Geometry check sheet. Reference: the model listing, model coordinates, mm. A direction names the side the tool comes from. Give positions to 0.01 mm unless a question says otherwise; leave off trailing zeros. Loops run counter-clockwise (first coordinate to the right, second up) from the corner with the lowest first, then second, coordinate; pieces in that order, holes last. Notation, with made-up numbers: (66, 88) -> (80, 88) arc R21 ccw to (80, 114) -> close; hole circle Ø5 at (32, 8). An arc over 180 degrees is marked (long way). Answer in a Markdown table with one row per item. Add a question column.
```python
from build123d import *

# Parameters (mm, degrees)
SKETCH1_W           = 20
SKETCH1_H           = 38
BOSS_EXTRUDE1_DEPTH = 3
SKETCH2_W           = 10
SKETCH2_H           = 3
CUT_EXTRUDE1_DEPTH  = 3
CUT_EXTRUDE2_DEPTH  = 3


with BuildPart() as part:
    # Sketch1 → Boss-Extrude1 (new body)
    with BuildSketch(Plane(origin=(0, 0, 0), x_dir=(0, 0, -1), z_dir=(1, 0, 0))):
        with Locations((10, 19)):
            Rectangle(SKETCH1_W, SKETCH1_H)
    extrude(amount=BOSS_EXTRUDE1_DEPTH)

    # Sketch2 → Cut-Extrude1 (cut)
    with BuildSketch(Plane(origin=(3, 0, 0), x_dir=(0, 0, -1), z_dir=(1, 0, 0))):
        with Locations((5, 36.5)):
            Rectangle(SKETCH2_W, SKETCH2_H)
        with Locations((5, 1.5)):
            Rectangle(SKETCH2_W, SKETCH2_H)
    extrude(amount=-CUT_EXTRUDE1_DEPTH, mode=Mode.SUBTRACT)

    # Sketch3 → Cut-Extrude2 (cut)
    with BuildSketch(Plane(origin=(3, 0, 0), x_dir=(0, 0, -1), z_dir=(1, 0, 0))):
        Polygon((3.45, 3), (3.45, 5.9), (2.05, 5.9), (2.05, 8.6), (3.45, 8.6), (3.45, 10.3), (6.55, 10.3), (6.55, 8.6), (7.95, 8.6), (7.95, 5.9), (6.55, 5.9), (6.55, 3), align=None)
        Polygon((6.55, 35), (6.55, 32.1), (7.95, 32.1), (7.95, 29.4), (6.55, 29.4), (6.55, 27.7), (3.45, 27.7), (3.45, 29.4), (2.05, 29.4), (2.05, 32.1), (3.45, 32.1), (3.45, 35), align=None)
    extrude(amount=-CUT_EXTRUDE2_DEPTH, mode=Mode.SUBTRACT)


solid = part.part
```
1. Material ranges on L1, parallel to Y at x = 0.55, z = -2.75; L2, parallel to Z at x = 0.8, y = 10; L3, parallel to Z at x = 0.6, y = 31, recorded low to high. Write a range as from..to.
2. Sectioned sample at B-B (z = -7.5). Enter the section's corners in (x, y).
3. Access from +Z, -Z, +X, -X, +Y, -Y to the whole of each face (thin tool, end or side, straight path). Record for faces 1 (the face through (2, 1, -10)), 2 (the face through (1, 0, -15)), 3 (the face through (2, 9, -6.55)), 4 (the face through (2, 8.6, -3)), 5 (the face through (2, 35, -8)).
4. Release check for a two-part mould opening along Y. For faces 6 (the face through (2, 27.7, -5)), 7 (the face through (2, 7, -2.05)), 8 (the face through (2, 4, -6.55)) record: released by +Y, released by -Y, zero draft, split by the parting line, or undercut.
5. Sectioned sample at A-A (y = 7). Enter the section's corners in (x, z), plus the area to 3 significant figures.
6. Sectioned sample at D-D (z = -4.5). Enter the section's corners in (x, y).
7. Gauge pin test, flat ends, axial feed: pin 1 Ø1.4 at (x, y) = (2, 28.5) entering from +Z; pin 2 Ø1.5 at (x, z) = (2, -3) entering from -Y; pin 3 Ø0.7 at (x, z) = (1, -7) entering from +Y. Record the tip position at first contact, or that the pin passes through.
Response:
| question | item | result |
|---|---|---|
| 1 | L1 | y = 3..5.9, 8.6..29.4, 32.1..35 |
| 1 | L2 | z = -20..-6.55, -3.45..0 |
| 1 | L3 | z = -20..-7.95, -2.05..0 |
| 2 | outline | (0, 3) -> (3, 3) -> (3, 5.9) -> (0, 5.9) -> close; (0, 8.6) -> (3, 8.6) -> (3, 29.4) -> (0, 29.4) -> close; (0, 32.1) -> (3, 32.1) -> (3, 35) -> (0, 35) -> close |
| 3 | face 1 | +Z, +X, -X, -Y |
| 3 | face 2 | +Z, -Z, +X, -X, -Y |
| 3 | face 3 | +X, -X, -Y |
| 3 | face 4 | +X, -X |
| 3 | face 5 | +Z, +X, -X, +Y |
| 4 | face 6 | released by +Y |
| 4 | face 7 | undercut |
| 4 | face 8 | zero draft |
| 5 | outline | (0, -20) -> (3, -20) -> (3, -7.95) -> (0, -7.95) -> close; (0, -2.05) -> (3, -2.05) -> (3, 0) -> (0, 0) -> close |
| 5 | area | 42.3 mm2 |
| 6 | outline | (0, 10.3) -> (3, 10.3) -> (3, 27.7) -> (0, 27.7) -> close |
| 7 | pin 1 | stops at z = 0 |
| 7 | pin 2 | stops at y = 3 |
| 7 | pin 3 | stops at y = 35 |
